The model under review builds one solid part; all positions refer to its coordinate system, in mm. A direction names the side the tool comes from. Round coordinates to 2 decimals unless told otherwise and drop trailing zeros. Loops run counter-clockwise (first coordinate to the right, second up) from the corner with the lowest first, then second, coordinate; pieces in that order, holes last. Notation, with made-up numbers: M 14,39.5 L 59,39.5 A33 ccw 59,78.5 Z; hole C 40,15.25 d7. An arc over 180 degrees is marked long. Use a Markdown table: item, result. Add a question column.
```python
from build123d import *

# Parameters (mm, degrees)
SKETCH1_R           = 2.75
SKETCH1_R_2         = 13
BOSS_EXTRUDE1_DEPTH = 13
FILLET1_R           = 1.7
FILLET2_R           = 0.5


with BuildPart() as part:
    # Sketch1 → Boss-Extrude1 (new body)
    with BuildSketch(Plane.XY):
        Polygon((40.027969698, 14.696983914), (27.527969698, 14.696983914), (27.527969698, 22.782770351), (25.113756136, 25.196983914), (-3.057816739, 25.196983914), (-5.472030302, 22.782770351), (-5.472030302, 14.696983914), (-17.972030302, 14.696983914), (-17.972030302, -15.803016086), (40.027969698, -15.803016086), align=None)
        with Locations((34.027969698, 8.196983914)):
            Circle(SKETCH1_R, mode=Mode.SUBTRACT)
        with Locations((34.027969698, -9.803016086)):
            Circle(SKETCH1_R, mode=Mode.SUBTRACT)
        with Locations((-11.972030302, -9.803016086)):
            Circle(SKETCH1_R, mode=Mode.SUBTRACT)
        with Locations((-11.972030302, 8.196983914)):
            Circle(SKETCH1_R, mode=Mode.SUBTRACT)
        with Locations((11.027969698, 8.196983914)):
            Circle(SKETCH1_R_2, mode=Mode.SUBTRACT)
    extrude(amount=BOSS_EXTRUDE1_DEPTH)

    # Fillet1
    fillet1_edges = [part.edges().sort_by_distance(p)[0] for p in [
        (-5.472030302, 14.696983914, 6.5),
        (27.527969698, 14.696983914, 6.5),
    ]]
    fillet(fillet1_edges, radius=FILLET1_R)

    # Fillet2
    fillet2_edges = [part.edges().sort_by_distance(p)[0] for p in [
        (40.027969698, -15.803016086, 6.5),
        (-17.972030302, -15.803016086, 6.5),
        (-17.972030302, 14.696983914, 6.5),
        (-5.472030302, 22.782770351, 6.5),
        (-3.057816739, 25.196983914, 6.5),
        (25.113756136, 25.196983914, 6.5),
        (27.527969698, 22.782770351, 6.5),
        (40.027969698, 14.696983914, 6.5),
    ]]
    fillet(fillet2_edges, radius=FILLET2_R)


solid = part.part
```
(1) Consider section D-D, the plane z = 8.25. Give the boundary of the cut face in (x, y).
(2) To check wall thickness, follow probe 1 along Y at (x, z) = (-9.5, 10.5); probe 2 along X at (y, z) = (-12, 1); probe 3 along X at (y, z) = (-9.5, 12). State the ranges of each line that lie inside material, in increasing order.
(3) Consider section A-A, the plane x = -10. Give the boundary of the cut face in (y, z).
(4) Consider section B-B, the plane y = 0. Give the boundary of the cut face in (x, z).
(5) Draft analysis for pull direction Y (two halves, no side actions). For faces 4 (the face through (26.336, 23.975, 6.409)), 5 (the face through (27.528, 19, 6)), 6 (the face through (36.65, 9.02, 6.41)), 7 (the face through (36.65, -8.98, 6.41)), state which applies: released by +Y, released by -Y, zero draft, split by the parting line, or undercut.
(6) For faces 1 (the face through (34, 14.697, 6)), 2 (the face through (11, -15.803, 6)), 3 (the face through (-12, 14.697, 6)), list the 3-axis set-ups (+Z, -Z, +X, -X, +Y, -Y) from which the entire face can be reached by the end or side of a thin tool; tool diameter is ignored.
(7) Consider section C-C, the plane x = 12. Give the boundary of the cut face in (y, z).
(8) Insertion check: pin 1 Ø5 at (x, z) = (-9, 2.5) entering from +Y; pin 2 Ø1 at (x, y) = (-9, -6.5) entering from -Z; pin 3 Ø7 at (y, z) = (19, 4) entering from -X; pin 4 Ø5 at (x, z) = (34, 9.5) entering from +Y. Each pin has a flat end and moves straight along its axis. Give the tip position at first contact, or say it passes through.
Found:
| question | item | result |
|---|---|---|
| 1 | outline | M -17.97,-15.3 A0.5 ccw -17.47,-15.8 L 39.53,-15.8 A0.5 ccw 40.03,-15.3 L 40.03,14.2 A0.5 ccw 39.53,14.7 L 29.23,14.7 A1.7 cw 27.53,16.4 L 27.53,22.58 A0.5 ccw 27.38,22.93 L 25.26,25.05 A0.5 ccw 24.91,25.2 L -2.85,25.2 A0.5 ccw -3.2,25.05 L -5.33,22.93 A0.5 ccw -5.47,22.58 L -5.47,16.4 A1.7 cw -7.17,14.7 L -17.47,14.7 A0.5 ccw -17.97,14.2 Z; hole C -11.97,-9.8 d5.5; hole C -11.97,8.2 d5.5; hole C 11.03,8.2 d26; hole C 34.03,-9.8 d5.5; hole C 34.03,8.2 d5.5 |
| 2 | probe 1 | y = -15.8 to -11.01, -8.6 to 6.99, 9.4 to 14.7 |
| 2 | probe 2 | x = -17.97 to -13.63, -10.32 to 32.37, 35.68 to 40.03 |
| 2 | probe 3 | x = -17.97 to -14.71, -9.24 to 31.29, 36.76 to 40.03 |
| 3 | outline | M -15.8,0 L -11.72,0 L -11.72,13 L -15.8,13 Z; M -7.89,0 L 6.28,0 L 6.28,13 L -7.89,13 Z; M 10.11,0 L 14.7,0 L 14.7,13 L 10.11,13 Z |
| 4 | outline | M -17.97,0 L 0.94,0 L 0.94,13 L -17.97,13 Z; M 21.12,0 L 40.03,0 L 40.03,13 L 21.12,13 Z |
| 5 | face 4 | released by +Y |
| 5 | face 5 | zero draft |
| 5 | face 6 | undercut |
| 5 | face 7 | undercut |
| 6 | face 1 | +Z, -Z, +X, +Y |
| 6 | face 2 | +Z, -Z, +X, -X, -Y |
| 6 | face 3 | +Z, -Z, -X, +Y |
| 7 | outline | M -15.8,0 L -4.77,0 L -4.77,13 L -15.8,13 Z; M 21.16,0 L 25.2,0 L 25.2,13 L 21.16,13 Z |
| 8 | pin 1 | stops at y = 14.84 |
| 8 | pin 2 | stops at z = 0 |
| 8 | pin 3 | stops at x = -5.73 |
| 8 | pin 4 | stops at y = 14.7 |
